Check sheet for the drawn part. Datum: minimum x, y, z corner. Units: mm. Coordinates: 2 decimals unless noted, no trailing zeros. Write each loop counter-clockwise with the first axis right and the second up, starting at its lowest first coordinate (ties: lowest second). Pieces come first, ordered by that corner, then holes. Notation, with made-up numbers: (18.25, 28.25) - (59.25, 28.25) arc R18 cw to (59.25, 53.25) - close; hole circle Ø10 at (44, 8.5). An arc over 180 degrees is marked (long way). Use one line per item in the form item = value. Start each with the question number.
1. Cross-section at A-A on x = 6. Record the boundary of the cut face in (y, z) (1 decimal).
2. Cross-section at B-B on y = 41. Record the boundary of the cut face in (x, z) (1 decimal), then the cut area to 3 significant figures.
3. Cross-section at C-C on z = 0.6. Give the number of separate pieces and of enclosed holes in the cut face, then the cut area to 3 significant figures.
4. Go/stop test with flat-tipped pins: pin 1 Ø1 at (x, z) = (52.5, 1) entering from +Y; pin 2 Ø1 at (x, z) = (10, 1.5) entering from -Y. Record where each tip stops, or that it passes through.
5. Scan lines: line 1 along X through (y, z) = (35, 1.35) (1 decimal); line 2 along X through (y, z) = (70, 2.65) (1 decimal); line 3 along X through (y, z) = (15, 2) (1 decimal). Record each from-to range of solid material in increasing order.
6. Cross-section at D-D on x = 53. Record the boundary of the cut face in (y, z) (1 decimal).
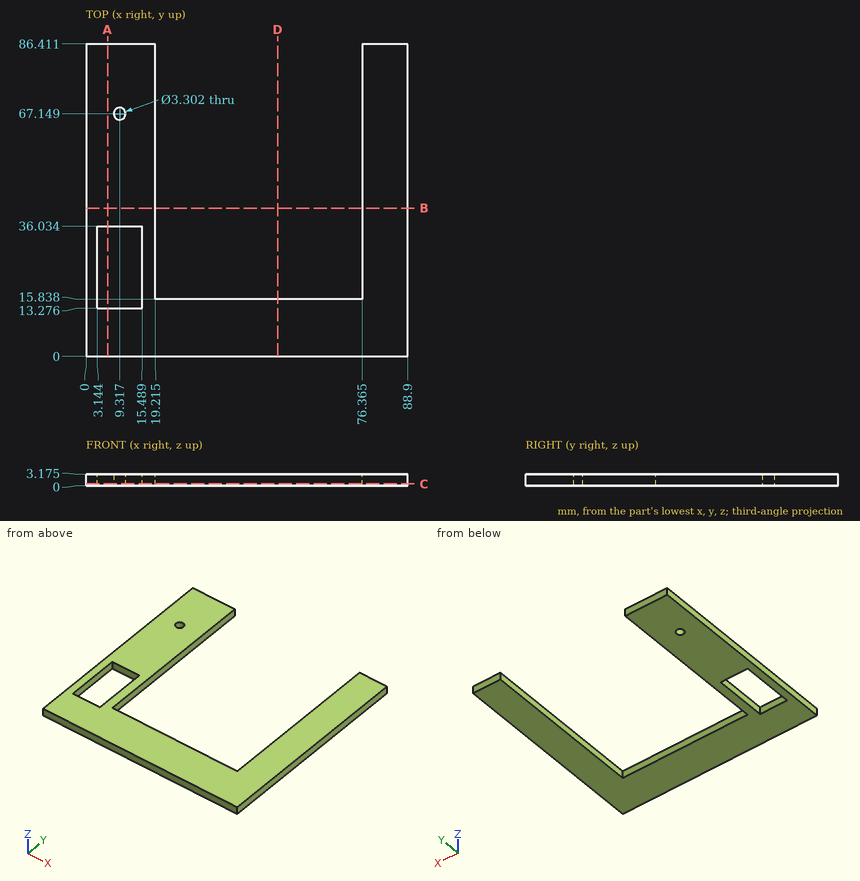
Final values:
q1.outline = (0, 0) - (13.3, 0) - (13.3, 3.2) - (0, 3.2) - close; (36, 0) - (86.4, 0) - (86.4, 3.2) - (36, 3.2) - close
q2.outline = (0, 0) - (19.2, 0) - (19.2, 3.2) - (0, 3.2) - close; (76.4, 0) - (88.9, 0) - (88.9, 3.2) - (76.4, 3.2) - close
q2.area = 101 mm²
q3.separate_pieces = 1
q3.enclosed_holes = 2
q3.area = 3,360 mm²
q4.pin_1 = 15.84
q4.pin_2 = 0
q5.line_1 = 0 to 3.1, 15.5 to 19.2, 76.4 to 88.9
q5.line_2 = 0 to 19.2, 76.4 to 88.9
q5.line_3 = 0 to 3.1, 15.5 to 88.9
q6.outline = (0, 0) - (15.8, 0) - (15.8, 3.2) - (0, 3.2) - close
